The figure shows three views and two pictorial views of one solid part (mm, origin at its lowest corner). Answer the questions. A direction names the side the tool comes from. Give positions to 0.01 mm unless a question says otherwise; leave off trailing zeros. Order: outer loops, then holes, each group sorted by start corner. A loop starts at its lowest first (then second) coordinate and runs counter-clockwise, first axis right, second up. Notation, with made-up numbers: (23.25, 35) -> (31.25, 35) arc R22 ccw to (31.25, 52) -> close; hole circle Ø7 at (64, -14.5). An arc over 180 degrees is marked (long way). One line per item, written item: value. Start each with the question number.
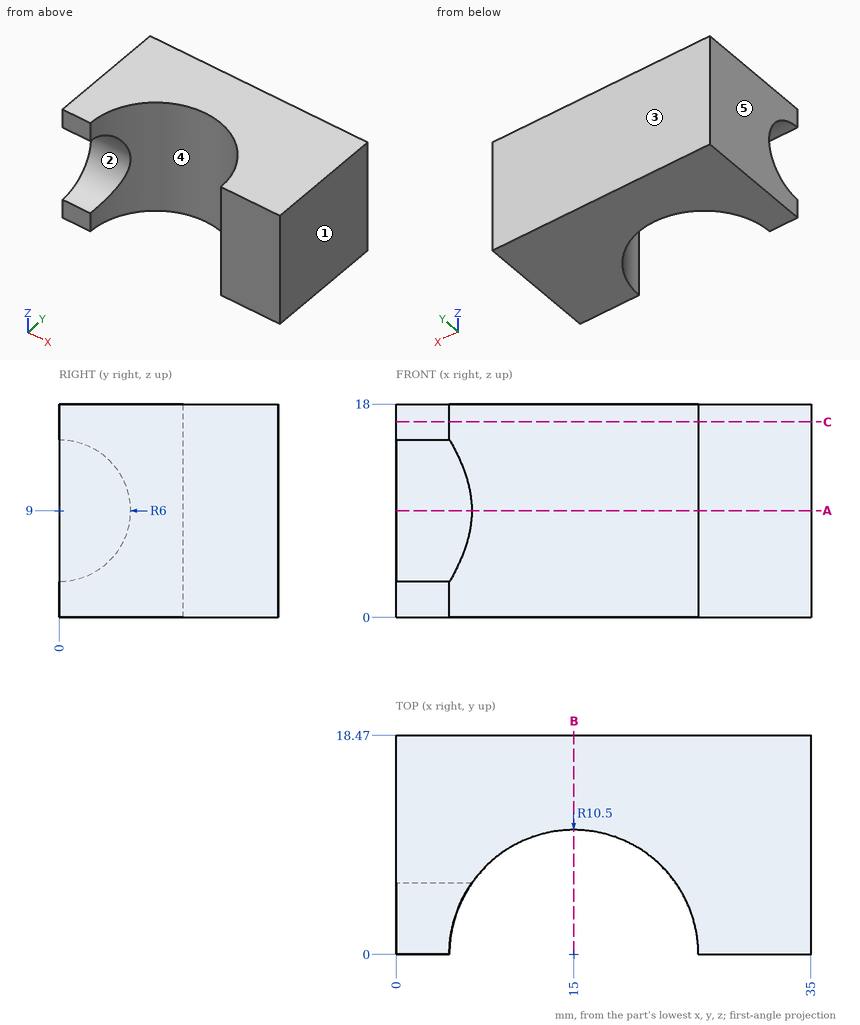
Item 1: Find the intervals of material crossed by line 1 (X direction, y = 1.5, z = 16.5); line 2 (X direction, y = 6.75, z = 7.75); line 3 (Y direction, x = 13, z = 2.5), in increasing order. Write a range as from..to.
Item 2: Find section B-B on x = 15. Write down the section's boundary in (y, z), then the cut area to 3 significant figures.
Item 3: A tool of negligible diameter and unlimited length cuts with its end or side. For the marked faces 1 and 2, from which of +Z, -Z, +X, -X, +Y, -Y can it reach the whole face along a straight path? Write none if from no direction.
Item 4: Find section C-C on z = 16.5. Write down the section's boundary in (x, y).
Item 5: For a pull along X with two mould halves and no side action, classify the marked faces 3, 4 and 5 as +X half, -X half, draft (parallel to the pull), parting line (faces both ways), or undercut.
Item 6: Find section A-A on z = 9. Write down the section's boundary in (x, y).
Checks:
1. line 1: 0..4.61, 25.39..35
1. line 2: 0..6.96, 23.04..35
1. line 3: 10.31..18.47
2. outline: (10.5, 0) -> (18.47, 0) -> (18.47, 18) -> (10.5, 18) -> close
2. area: 143 mm2
3. face 1: +Z, -Z, +X, +Y, -Y
3. face 2: -X, -Y
4. outline: (0, 0) -> (4.5, 0) arc R10.5 cw to (25.5, 0) -> (35, 0) -> (35, 18.47) -> (0, 18.47) -> close
5. face 3: draft
5. face 4: undercut
5. face 5: -X half
6. outline: (0, 6) -> (6.38, 6) arc R10.5 cw to (25.5, 0) -> (35, 0) -> (35, 18.47) -> (0, 18.47) -> close
